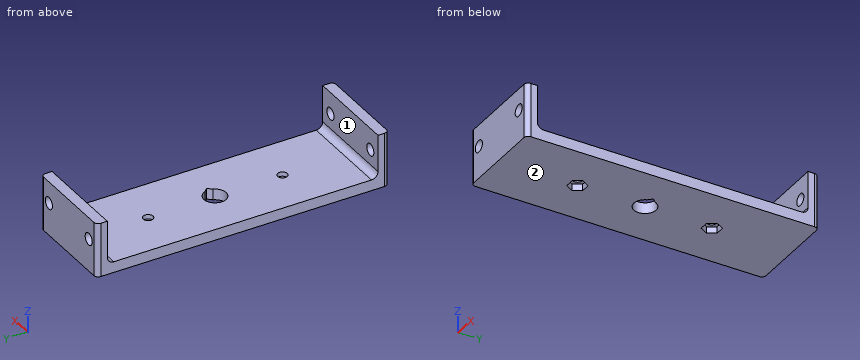
Autodesk Inventor part; units mm, degrees
ref_plane "YZ Plane" through (0, 0, 0) normal (1, 0, 0) x (0, 1, 0)
ref_plane "XZ Plane" through (0, 0, 0) normal (0, 1, 0) x (-1, 0, 0)
ref_plane "XY Plane" through (0, 0, 0) normal (0, 0, 1) x (1, 0, 0)
sketch "Sketch1" plane through (0, 0, 0) normal (0, 0, 1) x (1, 0, 0)
  circle A0 centre (0, 0) radius 2.25
  circle A1 centre (31, 0) radius 2.25
  circle A2 centre (0, 31) radius 2.25
  circle A3 centre (31, 31) radius 2.25
  circle A4 centre (15.5, 15.5) radius 5.125
  line L0 (-6, 37) -> (37, 37)
  line L1 (37, 37) -> (37, -6)
  line L2 (37, -6) -> (-6, -6)
  line L3 (-6, -6) -> (-6, 37)
  line L4 (-6, 37) -> (37, -6) construction
  line L5 (37, 37) -> (-6, -6) construction
  line L6 (-6, -6) -> (37, -6)
  line L7 (37, -6) -> (37, -52)
  line L8 (37, -52) -> (-6, -52)
  line L9 (-6, -52) -> (-6, -6)
  line L10 (-6, 15.5) -> (0, 15.5)
  line L11 (37, 37) -> (37, 83)
  line L12 (37, 83) -> (-6, 83)
  line L13 (-6, 83) -> (-6, 37)
  line L14 (20.625, 15.5) -> (22.125, 15.5)
  line L15 (22.125, 15.5) -> (20.2868, 17.3309)
  line L16 (22.125, 15.5) -> (20.2868, 13.6691)
  point P0 (37, 37)
  dimension "d3" = 4.5
  dimension "d5" = 31
  dimension "d6" = 10.25
  dimension "d7" = 43
  dimension "d8" = 43
  dimension "d9" = 67.5
  dimension "d10" = 31
  dimension "d44" = 1.5
extrude "Extrusion1" add sketch "Sketch1" against normal blind 5 contours A0 | A1 | A2 | A3 | L13 L12 L11 L0 | L0 L1 L2 L3 | L7 L8 L9 L2
sketch "Sketch2" plane through (0, 0, 0) normal (0, 0, 1) x (1, 0, 0)
  line L0 (37, -52) -> (-6, -52)
  line L1 (37, 83) -> (37, -52)
  line L2 (-6, -52) -> (37, -52)
  line L3 (37, -52) -> (37, -47)
  line L4 (37, -47) -> (-6, -47)
  line L5 (-6, -47) -> (-6, -52)
  line L6 (-6, 15.5) -> (0, 15.5)
  line L7 (37, 78) -> (-6, 78)
  line L8 (-6, 78) -> (37, 78)
  line L9 (-6, 83) -> (-6, -52)
  line L10 (-6, -52) -> (37, -52)
  line L11 (37, -52) -> (37, 83)
  line L12 (37, 83) -> (-6, 83)
  arc A0 (20.2868, 17.3309) -> (20.2868, 13.6691) centre (15.5, 15.5) ccw
  line L13 (22.125, 15.5) -> (20.2868, 13.6691)
  line L14 (20.2868, 17.3309) -> (22.125, 15.5)
  point P0 (0, 0)
  point P1 (37, 37)
  point P2 (-6, 37)
  point P3 (-6, 78)
  point P4 (37, 78)
  dimension "d13" = 5
extrude "Extrusion2" add sketch "Sketch2" along normal blind 20 contours L0 L5 L4 L1 | L7 L9 L12 L1
sketch "Sketch3" plane through (-6, -47, 0) normal (0, 1, 0) x (1, 0, 0)
  circle A0 centre (6, -10) radius 2.75
  circle A1 centre (37, -10) radius 2.75
  line L0 (0, 5) -> (0, -20)
  line L1 (0, 0) -> (0, -20)
  line L2 (43, 0) -> (43, -20)
  line L3 (0, 5) -> (43, 5)
  line L4 (0, 0) -> (43, 0)
  line L5 (43, 5) -> (0, 5)
  line L6 (6, -10) -> (6, -15) construction
  arc A2 (8.75, -10) -> (3.25, -10) centre (6, -10) ccw
  line L7 (21.5, 0) -> (21.5, -10)
  arc A3 (39.75, -10) -> (34.25, -10) centre (37, -10) ccw
  line L8 (6, -10) -> (6, -5) construction
  line L9 (3.25, -10) -> (3.25, -5)
  line L10 (8.75, -5) -> (8.75, -10)
  arc A4 (3.25, -10) -> (8.75, -10) centre (6, -10) ccw
  arc A5 (8.75, -5) -> (3.25, -5) centre (6, -5) ccw
  line L11 (37, -10) -> (37, -5) construction
  line L12 (39.75, -10) -> (39.75, -5)
  line L13 (34.25, -5) -> (34.25, -10)
  arc A6 (39.75, -5) -> (34.25, -5) centre (37, -5) ccw
  point P0 (6, 0)
  point P1 (0, -10)
  point P2 (6, -12.5)
  point P3 (6, -7.5)
  point P4 (39.75, -10)
  point P5 (3.25, -10)
  dimension "d16" = 5.5
  dimension "d17" = 31
  dimension "d23" = 6
  dimension "d38" = 15
  dimension "d39" = 5
  dimension "d43" = 5
extrude "Extrusion3" [suppressed]
sketch "Sketch8" plane through (-6, 83, 0) normal (0, -1, 0) x (1, 0, 0)
  circle A0 centre (6, 10) radius 2.75
  circle A1 centre (37, 10) radius 2.75
  point P0 (6, 0)
extrude "Extrusion8" cut sketch "Sketch8" along normal blind 160.5
fillet "Fillet2" [suppressed]
sketch "Sketch9" plane through (0, 0, -5) normal (0, 0, -1) x (-1, 0, 0)
  circle A0 centre (-15.235, 46.5) radius 2.25
  circle A1 centre (-15.235, -15.5) radius 2.25
  line L0 (-37, 83) -> (-37, -52)
  line L1 (-37, -52) -> (6, -52)
  line L2 (6, -52) -> (6, 83)
  line L3 (6, 83) -> (-37, 83)
  arc A2 (-20.2868, 13.6691) -> (-20.2868, 17.3309) centre (-15.5, 15.5) ccw
  line L4 (-20.2868, 13.6691) -> (-22.125, 15.5)
  line L5 (-22.125, 15.5) -> (-20.2868, 17.3309)
  point P0 (0, 0)
  dimension "d45" = 62
  dimension "d46" = 31
  dimension "d49" = 4.5
extrude "Extrusion9" cut sketch "Sketch9" against normal blind 10 contours A0 | A1
sketch "Sketch10" plane through (0, 0, -5) normal (0, 0, 1) x (1, 0, 0)
  circle A0 centre (15.235, -15.5) radius 2.25
  circle A1 centre (15.235, 46.5) radius 2.25
  line L0 (-6, -47) -> (37, -47)
  line L1 (37, -47) -> (37, 78)
  line L2 (37, 78) -> (-6, 78)
  line L3 (-6, 78) -> (-6, -47)
  arc A2 (20.2868, 17.3309) -> (20.2868, 13.6691) centre (15.5, 15.5) ccw
  line L4 (11.286, 46.5) -> (13.2605, 49.92)
  line L5 (13.2605, 49.92) -> (17.2096, 49.92)
  line L6 (17.2096, 49.92) -> (19.1841, 46.5)
  line L7 (19.1841, 46.5) -> (17.2096, 43.08)
  line L8 (17.2096, 43.08) -> (13.2605, 43.08)
  line L9 (13.2605, 43.08) -> (11.286, 46.5)
  line L10 (10.9973, 46.5) -> (13.1162, 50.17)
  line L11 (13.1162, 50.17) -> (17.3539, 50.17)
  line L12 (17.3539, 50.17) -> (19.4728, 46.5)
  line L13 (19.4728, 46.5) -> (17.3539, 42.83)
  line L14 (17.3539, 42.83) -> (13.1162, 42.83)
  line L15 (13.1162, 42.83) -> (10.9973, 46.5)
  line L16 (15.5, 15.5) -> (12.1559, 15.5)
  circle A3 centre (15.235, -15.5) radius 2.25
  line L17 (11.286, -15.5) -> (13.2605, -18.92)
  line L18 (13.2605, -18.92) -> (17.2096, -18.92)
  line L19 (17.2096, -18.92) -> (19.1841, -15.5)
  line L20 (19.1841, -15.5) -> (17.2096, -12.08)
  line L21 (17.2096, -12.08) -> (13.2605, -12.08)
  line L22 (13.2605, -12.08) -> (11.286, -15.5)
  line L23 (10.9973, -15.5) -> (13.1162, -19.17)
  line L24 (13.1162, -19.17) -> (17.3539, -19.17)
  line L25 (17.3539, -19.17) -> (19.4728, -15.5)
  line L26 (19.4728, -15.5) -> (17.3539, -11.83)
  line L27 (17.3539, -11.83) -> (13.1162, -11.83)
  line L28 (13.1162, -11.83) -> (10.9973, -15.5)
  line L29 (22.125, 15.5) -> (20.2868, 13.6691)
  line L30 (20.2868, 17.3309) -> (22.125, 15.5)
  point P0 (0, 0)
  dimension "d50" = 6.84
  dimension "d51" = 0.25
extrude "M4_hex_neg" cut sketch "Sketch10" along normal blind 3 contours A0 | A1 | L4 L5 L6 L7 L8 L9 | L10 L11 L12 L13 L14 L15 | L22 L21 L20 L19 L18 L17 | L28 L27 L26 L25 L24 L23
fillet "Fillet3" radius 3 2 edges at (15.5, 78, 0) (15.5, -47, 0)
fillet "Fillet4" radius 2 4 edges at (37, -52, 7.5) (37, 83, 7.5) (-6, 83, 7.5) (-6, -52, 7.5)
properties part number "motor_holder"
The model under review builds one solid part; all positions refer to its coordinate system, in mm. Face numbers are marked on the shaded views. A direction names the side the tool comes from. Round coordinates to 2 decimals unless told otherwise and drop trailing zeros. Order: outer loops, then holes, each group sorted by start corner. A loop starts at its lowest first (then second) coordinate and runs counter-clockwise, first axis right, second up. Notation, with made-up numbers: (-6.75, 23.25) -> (12.25, 23.25) arc R9 ccw to (12.25, 35.25) -> close; hole circle Ø10 at (78.25, 5.25). An arc over 180 degrees is marked (long way). Use CSV: the item, a comma, the result in double quotes. Start each with the question number.
(1) Consider section C-C on x = 31. Write out the cut boundary in (y, z), and give its area (3 significant figures).
(2) Insertion check: pin 1 (12 mm diameter, centred on x = 15.5, y = 15.5, fed in from +Z); pin 2 (7 mm diameter, centred on x = 31, z = 10, fed in from -Y). Each pin has a flat end and moves straight along its axis. Give the tip position at first contact, or say it passes through.
(3) Consider section A-A on z = 5.25. Write out the cut boundary in (x, y).
(4) Consider section B-B on x = 15.5. State how many separate pieces and enclosed holes the cut face has, and give its area (3 significant figures).
(5) Tool access review of the marked faces 1 and 2: name each direction out of +Z, -Z, +X, -X, +Y, -Y from which nothing blocks a thin tool from reaching the whole face with its end or side.
(6) Wall thickness on probe 1 along Y at (x, z) = (15.5, -2.75) (3 decimals); probe 2 along X at (y, z) = (-49.2, 10); probe 3 along Y at (x, z) = (15.5, -1.6) (3 decimals): over which ranges is each line inside the solid? List them lowest first. Write a range as from..to.
(7) Consider section D-D on z = 11.5. Write out the cut boundary in (x, y), and give its area (3 significant figures).
Responses:
1,outline,"(-52, -5) -> (83, -5) -> (83, 7.25) -> (78, 7.25) -> (78, 3) arc R3 cw to (75, 0) -> (-44, 0) arc R3 cw to (-47, 3) -> (-47, 7.25) -> (-52, 7.25) -> close; (-52, 12.75) -> (-47, 12.75) -> (-47, 20) -> (-52, 20) -> close; (78, 12.75) -> (83, 12.75) -> (83, 20) -> (78, 20) -> close"
1,area,"824 mm²"
2,pin 1,"z = 0"
2,pin 2,"y = -52"
3,outline,"(-6, -50) arc R2 ccw to (-4, -52) -> (35, -52) arc R2 ccw to (37, -50) -> (37, -47) -> (-6, -47) -> close; (-6, 78) -> (37, 78) -> (37, 81) arc R2 ccw to (35, 83) -> (-4, 83) arc R2 ccw to (-6, 81) -> close"
4,separate pieces,"4"
4,enclosed holes,"0"
4,area,"766 mm²"
5,face 1,"+Z, +X, -X"
5,face 2,"-Z, +X, -X, +Y, -Y"
6,probe 1,"-52..-19.17, -11.83..10.375, 20.625..42.83, 50.17..83"
6,probe 2,"-6..-2.75, 2.75..28.25, 33.75..37"
6,probe 3,"-52..-17.734, -13.266..10.375, 20.625..44.266, 48.734..83"
7,outline,"(-6, -50) arc R2 ccw to (-4, -52) -> (-2.3, -52) -> (-2.3, -47) -> (-6, -47) -> close; (-6, 78) -> (-2.3, 78) -> (-2.3, 83) -> (-4, 83) arc R2 ccw to (-6, 81) -> close; (2.3, -52) -> (28.7, -52) -> (28.7, -47) -> (2.3, -47) -> close; (2.3, 78) -> (28.7, 78) -> (28.7, 83) -> (2.3, 83) -> close; (33.3, -52) -> (35, -52) arc R2 ccw to (37, -50) -> (37, -47) -> (33.3, -47) -> close; (33.3, 78) -> (37, 78) -> (37, 81) arc R2 ccw to (35, 83) -> (33.3, 83) -> close"
7,area,"334 mm²"
